For this review, take the finished solid that the model builds, in its own axes (mm). A direction names the side the tool comes from. Round coordinates to 2 decimals unless told otherwise and drop trailing zeros. Loops run counter-clockwise (first coordinate to the right, second up) from the corner with the lowest first, then second, coordinate; pieces in that order, holes last.
1. Consider section C-C on z = -33.5. State the section outline as (x, y) points.
2. Clearance check with a flat-ended pin moving along its axis: pin 1 Ø12 at (x, z) = (94, -111.5) entering from -Y. State where the tip first meets the part, or that it passes through.
3. Draft analysis for pull direction Z (two halves, no side actions). For faces 1 (the flat face through (91.43, 11.51, -87.88)), 2 (the flat face through (10, 11.3, -10)), 3 (the flat face through (79, 12, -81)), state which applies: released by +Z, released by -Z, zero draft, split by the parting line, or undercut.
4. Consider section A-A on y = 6.25. State the section outline as (x, z) points, then the cut area to 3 significant figures.
5. To check wall thickness, follow line 1 along Z through (x, y) = (30.5, 11.75); line 2 along X through (y, z) = (7.25, -56); line 3 along Z through (x, y) = (74, 7.5). State the ranges of each line that lie inside material, in increasing order.
6. Tool access review of faces 4 (the flat face through (2, 5, -81)), 5 (the flat face through (35.43, 11.51, -54.8)): name each direction out of +Z, -Z, +X, -X, +Y, -Y from which nothing blocks a thin tool from reaching the whole face with its end or side.
7. Consider section D-D on x = 133. State the section outline as (y, z) points.
8. Consider section B-B on x = 48. State the section outline as (y, z) points.
from build123d import *

# Parameters (mm, degrees)
BOSS_EXTRUDE1_DEPTH = 12
SKETCH5_W           = 155.5
SKETCH5_H           = 155.5
CUT_EXTRUDE3_DEPTH  = 11
CUT_EXTRUDE4_DEPTH  = 11


with BuildPart() as part:
    # Sketch1 → Boss-Extrude1 (new body)
    with BuildSketch(Plane(origin=(0, 0, 0), x_dir=(1, 0, 0), z_dir=(0, 1, 0))):
        Polygon((20, 159.5), (0, 139.5), (0, 20), (20, 0), (139.5, 0), (159.5, 20), (159.5, 139.5), (139.5, 159.5), align=None)
    extrude(amount=BOSS_EXTRUDE1_DEPTH)

    # Sketch5 → Cut-Extrude3 (cut)
    with BuildSketch(Plane.XZ):
        with Locations((79.75, -79.75)):
            Rectangle(SKETCH5_W, SKETCH5_H)
    extrude(amount=-CUT_EXTRUDE3_DEPTH, mode=Mode.SUBTRACT)

    # Sketch7 → Cut-Extrude4 (cut)
    with BuildSketch(Plane(origin=(0, 12, 0), x_dir=(1, 0, 0), z_dir=(0, 1, 0))):
        Polygon((139.5, 123.726497308), (139.5, 135.273502692), (129.5, 141.047005384), (119.5, 135.273502692), (119.5, 123.726497308), (129.5, 117.952994616), align=None)
        Polygon((106.5, 123.726497308), (106.5, 135.273502692), (96.5, 141.047005384), (86.5, 135.273502692), (86.5, 123.726497308), (96.5, 117.952994616), align=None)
        Polygon((73.5, 123.726497308), (73.5, 135.273502692), (63.5, 141.047005384), (53.5, 135.273502692), (53.5, 123.726497308), (63.5, 117.952994616), align=None)
        Polygon((40.5, 123.726497308), (40.5, 135.273502692), (30.5, 141.047005384), (20.5, 135.273502692), (20.5, 123.726497308), (30.5, 117.952994616), align=None)
        Polygon((106.5, 90.726497308), (106.5, 102.273502692), (96.5, 108.047005384), (86.5, 102.273502692), (86.5, 90.726497308), (96.5, 84.952994616), align=None)
        Polygon((73.5, 90.726497308), (73.5, 102.273502692), (63.5, 108.047005384), (53.5, 102.273502692), (53.5, 90.726497308), (63.5, 84.952994616), align=None)
        Polygon((40.5, 90.726497308), (40.5, 102.273502692), (30.5, 108.047005384), (20.5, 102.273502692), (20.5, 90.726497308), (30.5, 84.952994616), align=None)
        Polygon((106.5, 57.726497308), (106.5, 69.273502692), (96.5, 75.047005384), (86.5, 69.273502692), (86.5, 57.726497308), (96.5, 51.952994616), align=None)
        Polygon((73.5, 57.726497308), (73.5, 69.273502692), (63.5, 75.047005384), (53.5, 69.273502692), (53.5, 57.726497308), (63.5, 51.952994616), align=None)
        Polygon((40.5, 57.726497308), (40.5, 69.273502692), (30.5, 75.047005384), (20.5, 69.273502692), (20.5, 57.726497308), (30.5, 51.952994616), align=None)
        Polygon((106.5, 24.726497308), (106.5, 36.273502692), (96.5, 42.047005384), (86.5, 36.273502692), (86.5, 24.726497308), (96.5, 18.952994616), align=None)
        Polygon((73.5, 24.726497308), (73.5, 36.273502692), (63.5, 42.047005384), (53.5, 36.273502692), (53.5, 24.726497308), (63.5, 18.952994616), align=None)
        Polygon((40.5, 24.726497308), (40.5, 36.273502692), (30.5, 42.047005384), (20.5, 36.273502692), (20.5, 24.726497308), (30.5, 18.952994616), align=None)
        Polygon((139.5, 90.726497308), (139.5, 102.273502692), (129.5, 108.047005384), (119.5, 102.273502692), (119.5, 90.726497308), (129.5, 84.952994616), align=None)
        Polygon((139.5, 57.726497308), (139.5, 69.273502692), (129.5, 75.047005384), (119.5, 69.273502692), (119.5, 57.726497308), (129.5, 51.952994616), align=None)
        Polygon((139.5, 24.726497308), (139.5, 36.273502692), (129.5, 42.047005384), (119.5, 36.273502692), (119.5, 24.726497308), (129.5, 18.952994616), align=None)
    extrude(amount=-CUT_EXTRUDE4_DEPTH, mode=Mode.SUBTRACT)


solid = part.part
Resolved:
1. outline: (0, 0) - (2, 0) - (2, 11) - (20.5, 11) - (20.5, 12) - (0, 12) - close; (40.5, 11) - (53.5, 11) - (53.5, 12) - (40.5, 12) - close; (73.5, 11) - (86.5, 11) - (86.5, 12) - (73.5, 12) - close; (106.5, 11) - (119.5, 11) - (119.5, 12) - (106.5, 12) - close; (139.5, 11) - (157.5, 11) - (157.5, 0) - (159.5, 0) - (159.5, 12) - (139.5, 12) - close
2. pin 1: stops at y = 11
3. face 1: undercut
3. face 2: released by +Z
3. face 3: zero draft
4. outline: (0, -139.5) - (2, -141.5) - (2, -18) - (0, -20) - close; (18, -157.5) - (20, -159.5) - (139.5, -159.5) - (141.5, -157.5) - close; (18, -2) - (141.5, -2) - (139.5, 0) - (20, 0) - close; (157.5, -141.5) - (159.5, -139.5) - (159.5, -20) - (157.5, -18) - close
4. area: 972 mm2
5. line 1: z = -159.5 to -141.05, -117.95 to -108.05, -84.95 to -75.05, -51.95 to -42.05, -18.95 to 0
5. line 2: x = 0 to 2, 157.5 to 159.5
5. line 3: z = -159.5 to -157.5, -2 to 0
6. face 4: +Z, -Z, -Y
6. face 5: +Y, -Y
7. outline: (0, -159.5) - (12, -159.5) - (12, -139.03) - (11, -139.03) - (11, -157.5) - (0, -157.5) - close; (0, -2) - (11, -2) - (11, -20.97) - (12, -20.97) - (12, 0) - (0, 0) - close; (11, -119.97) - (12, -119.97) - (12, -106.03) - (11, -106.03) - close; (11, -86.97) - (12, -86.97) - (12, -73.03) - (11, -73.03) - close; (11, -53.97) - (12, -53.97) - (12, -40.03) - (11, -40.03) - close
8. outline: (0, -159.5) - (12, -159.5) - (12, 0) - (0, 0) - (0, -2) - (11, -2) - (11, -157.5) - (0, -157.5) - close
